The model under review builds one solid part; all positions refer to its coordinate system, in mm. Give positions to 0.01 mm unless a question says otherwise; leave off trailing zeros. Write each loop counter-clockwise with the first axis right and the second up, starting at its lowest first coordinate (ties: lowest second). Pieces come first, ordered by that corner, then holes. Notation, with made-up numbers: (75.5, -27) - (89.5, -27) arc R20 ccw to (89.5, -17) - close; hole circle Ø4 at (49, 53.25). An arc over 180 degrees is marked (long way). Write item = value, one per line.
```python
from build123d import *

# Parameters (mm, degrees)
F0_R     = 44.45
F1_DEPTH = 6.35
F3_DEPTH = 0.254


# Not quite as in the source:
# - ends of sketch curves that miss each other by under 0.0002 mm in the source are joined


with BuildPart() as f1:
    # F0 (on Top) → F1 (new body)
    with BuildSketch(Plane.XY):
        Circle(F0_R)
    extrude(amount=F1_DEPTH)

    # F2 (on face) → F3 (cut)
    with BuildSketch(Plane.XY.offset(6.35)):
        with BuildLine():
            Line((5.6039993651, 23.2917912652), (5.6039993651, 26.2641511811))
            Line((5.6039993651, 26.2641511811), (-3.5374157604, 26.2641511811))
            ThreePointArc((-3.5374157604, 26.2641511811), (-6.1724008767, 25.2877017598), (-7.2804156008, 22.7052797559))
            Line((-7.2804156008, 22.7052797559), (-7.2804156008, 14.3152289093))
            ThreePointArc((-7.2804156008, 14.3152289093), (-6.4557803762, 12.2478717336), (-4.4346582144, 11.3156409934))
            ThreePointArc((-4.4346582144, 11.3156409934), (1.3092272973, 11.2673019991), (7.0349466987, 11.7263169959))
            Line((7.0349466987, 11.7263169959), (7.0961336605, 12.2146336362))
            Line((7.0961336605, 12.2146336362), (7.0961336605, 19.8627323627))
            Line((7.0961336605, 19.8627323627), (0, 19.8627323627))
            Line((0, 19.8627323627), (0, 17.358450219))
            Line((0, 17.358450219), (2.9400843196, 17.3616167158))
            Line((2.9400843196, 17.3616167158), (2.9400843196, 14.1317071393))
            Line((2.9400843196, 14.1317071393), (0, 14.1317071393))
            Line((0, 14.1317071393), (-2.2346060723, 14.1317071393))
            ThreePointArc((-2.2346060723, 14.1317071393), (-2.7898678793, 14.3800667532), (-3.1146267429, 14.8943914101))
            ThreePointArc((-3.1146267429, 14.8943914101), (-3.2355914853, 15.5005322545), (-3.2674165577, 16.1178055789))
            Line((-3.2674165577, 16.1178055789), (-3.1592417437, 21.2145812126))
            ThreePointArc((-3.1592417437, 21.2145812126), (-3.1837866635, 21.575252567), (-3.1439608429, 21.9345577061))
            ThreePointArc((-3.1439608429, 21.9345577061), (-3.117530452, 22.198564373), (-3.1439608429, 22.4625710398))
            ThreePointArc((-3.1439608429, 22.4625710398), (-3.0817290753, 22.8241742068), (-2.7919525746, 23.0492502451))
            ThreePointArc((-2.7919525746, 23.0492502451), (-2.1422008965, 23.2306538656), (-1.4703774561, 23.2917912652))
            Line((-1.4703774561, 23.2917912652), (5.6039993651, 23.2917912652))
        make_face()
        with BuildLine():
            Line((-3.1592417437, 21.2145812126), (-3.1439608429, 21.9345577061))
            ThreePointArc((-3.1439608429, 21.9345577061), (-3.1837866635, 21.575252567), (-3.1592417437, 21.2145812126))
        make_face()
        Polygon((7.0961336605, 12.2146336362), (7.0349466987, 11.7263169959), (7.0961336605, 10.9925279394), (7.0961336605, 0.9659290663), (19.5016358048, 0.9659290663), (19.5016358048, 12.2146336362), align=None)
        Polygon((7.0961336605, 0.9659290663), (7.0961336605, 10.9925279394), (2.7143813204, 10.9925279394), (2.7143813204, 2.2997791572), (-2.7398910557, 10.9925279394), (-7.300500758, 10.9925279394), (-7.2804156008, 0), (-7.2804156008, -3.8537723012), (-6.2781353481, -3.8537723012), (-3.1410043308, -3.8537723012), (-3.1410043308, 4.7863919603), (2.6191033489, -3.8537723012), (7.0961336605, -3.8537723012), align=None)
        Polygon((-7.2804156008, 0), (-7.300500758, 10.9925279394), (-7.2804156008, 13.206558302), (-18.3086954057, 13.206558302), (-18.3086954057, 0), align=None)
        with BuildLine():
            Line((0, -7.2983574902), (6.6179535352, -7.2983574902))
            Line((6.6179535352, -7.2983574902), (6.6179535352, -4.2878086955))
            Line((6.6179535352, -4.2878086955), (-2.2489061664, -4.2878086955))
            ThreePointArc((-2.2489061664, -4.2878086955), (-4.0568875501, -4.6442817118), (-5.5942512015, -5.6603440615))
            ThreePointArc((-5.5942512015, -5.6603440615), (-6.1507192567, -6.4794007942), (-6.3533238135, -7.4486592847))
            Line((-6.3533238135, -7.4486592847), (-6.3533238135, -16.6105034737))
            ThreePointArc((-6.3533238135, -16.6105034737), (-5.8759308245, -17.9913268961), (-4.6476325952, -18.782440573))
            Line((-4.6476325952, -18.782440573), (-3.7075637703, -19.2863568686))
            Line((-3.7075637703, -19.2863568686), (3.3881619917, -19.303988614))
            Line((3.3881619917, -19.303988614), (6.6293859856, -18.9052186906))
            Line((6.6293859856, -18.9052186906), (6.593650474, -16.0276701207))
            Line((6.593650474, -16.0276701207), (0, -16.3928680122))
            ThreePointArc((0, -16.3928680122), (-0.7145080017, -16.4126398372), (-1.4290160034, -16.3928680122))
            ThreePointArc((-1.4290160034, -16.3928680122), (-2.080113152, -16.0523673946), (-2.251843689, -15.3379607946))
            Line((-2.251843689, -15.3379607946), (-2.251843689, -8.4599647671))
            ThreePointArc((-2.251843689, -8.4599647671), (-2.0899663646, -7.8730095416), (-1.6501033679, -7.4520092458))
            ThreePointArc((-1.6501033679, -7.4520092458), (-0.8286208401, -7.3368533365), (0, -7.2983574902))
        make_face()
        with BuildLine():
            Line((3.3881619917, -19.303988614), (-3.7075637703, -19.2863568686))
            Line((-3.7075637703, -19.2863568686), (-12.6563319936, -19.2641206086))
            Line((-12.6563319936, -19.2641206086), (-12.8377182409, -19.2641206086))
            Line((-12.8377182409, -19.2641206086), (-12.9873463884, -18.6591409147))
            ThreePointArc((-12.9873463884, -18.6591409147), (-13.1098010784, -17.8878071535), (-13.4031539783, -17.1640012413))
            ThreePointArc((-13.4031539783, -17.1640012413), (-13.5725884432, -16.8395453931), (-13.7304924428, -16.5093243122))
            ThreePointArc((-13.7304924428, -16.5093243122), (-14.0521811274, -16.0543913958), (-14.5178735256, -15.7484859228))
            ThreePointArc((-14.5178735256, -15.7484859228), (-15.086809482, -15.6747136098), (-15.6148988754, -15.8988833427))
            ThreePointArc((-15.6148988754, -15.8988833427), (-16.1466107031, -16.4449553577), (-16.5172908455, -17.1109195799))
            ThreePointArc((-16.5172908455, -17.1109195799), (-16.7501696159, -17.7330376736), (-16.9609729201, -18.3629784733))
            ThreePointArc((-16.9609729201, -18.3629784733), (-17.0934179213, -18.9312665088), (-17.1379111707, -19.5130854845))
            Line((-17.1379111707, -19.5130854845), (-17.1379111707, -19.8522191495))
            Line((-17.1379111707, -19.8522191495), (-19.3871874362, -19.8522191495))
            Line((-19.3871874362, -19.8522191495), (-19.3871874362, -22.8021256626))
            Line((-19.3871874362, -22.8021256626), (-17.0194374538, -22.8021256626))
            Line((-17.0194374538, -22.8021256626), (-17.0194374538, -23.2551640704))
            ThreePointArc((-17.0194374538, -23.2551640704), (-16.9093551317, -23.6838787474), (-16.7950224131, -24.1114795208))
            ThreePointArc((-16.7950224131, -24.1114795208), (-16.7338426372, -24.3328635786), (-16.6711639613, -24.5538279414))
            ThreePointArc((-16.6711639613, -24.5538279414), (-16.4738073507, -25.0326716474), (-16.1757338792, -25.4562199116))
            ThreePointArc((-16.1757338792, -25.4562199116), (-15.9267297619, -25.732701627), (-15.6729177634, -26.0047763574))
            ThreePointArc((-15.6729177634, -26.0047763574), (-14.9718242273, -26.3117655956), (-14.2623546636, -26.0246637372))
            ThreePointArc((-14.2623546636, -26.0246637372), (-13.7772653209, -25.4368959002), (-13.4154763073, -24.7661564499))
            ThreePointArc((-13.4154763073, -24.7661564499), (-13.2751868701, -24.4473909933), (-13.1237693131, -24.1337586194))
            ThreePointArc((-13.1237693131, -24.1337586194), (-12.9090296801, -23.5454392253), (-12.837051295, -22.9233042467))
            Line((-12.837051295, -22.9233042467), (-12.8377182409, -22.622095421))
            Line((-12.8377182409, -22.622095421), (0.5678676759, -22.592412358))
            Line((0.5678676759, -22.592412358), (12.5019904939, -22.6220667474))
            Line((12.5019904939, -22.6220667474), (12.5135298725, -22.622095421))
            Line((12.5135298725, -22.622095421), (12.6259239413, -22.622095421))
            Line((12.6259239413, -22.622095421), (12.6259239413, -22.8433404118))
            ThreePointArc((12.6259239413, -22.8433404118), (12.6900931034, -23.3765945805), (12.878936831, -23.8794024329))
            ThreePointArc((12.878936831, -23.8794024329), (13.1121897024, -24.7032143779), (13.6001783309, -25.4067341867))
            Line((13.6001783309, -25.4067341867), (13.7601625174, -25.5711600184))
            ThreePointArc((13.7601625174, -25.5711600184), (14.0077931702, -25.8774350672), (14.3499616533, -26.0724890977))
            ThreePointArc((14.3499616533, -26.0724890977), (14.8915415981, -26.1493664388), (15.4228175364, -26.0191172952))
            ThreePointArc((15.4228175364, -26.0191172952), (15.5930961418, -25.9161088082), (15.7359875739, -25.7775895298))
            ThreePointArc((15.7359875739, -25.7775895298), (16.5550328697, -24.4671777543), (17.0114282519, -22.9907911271))
            Line((17.0114282519, -22.9907911271), (17.0942133791, -22.5096959621))
            Line((17.0942133791, -22.5096959621), (19.0433021635, -22.5096959621))
            Line((19.0433021635, -22.5096959621), (19.0433021635, -19.4356404245))
            Line((19.0433021635, -19.4356404245), (17.0150939375, -19.4110530503))
            Line((17.0150939375, -19.4110530503), (17.0150939375, -19.0368138024))
            ThreePointArc((17.0150939375, -19.0368138024), (16.989674065, -18.7347053505), (16.9141292572, -18.4410922229))
            Line((16.9141292572, -18.4410922229), (16.690004617, -17.6846757531))
            ThreePointArc((16.690004617, -17.6846757531), (16.407642716, -17.0034564681), (15.9896202385, -16.3959655911))
            ThreePointArc((15.9896202385, -16.3959655911), (15.6603689447, -16.0642729564), (15.2857392253, -15.7848467735))
            ThreePointArc((15.2857392253, -15.7848467735), (14.6670179234, -15.6398096454), (14.0927875351, -15.9120435136))
            Line((14.0927875351, -15.9120435136), (13.9366754533, -16.0662262266))
            ThreePointArc((13.9366754533, -16.0662262266), (13.2239743808, -16.988100564), (12.7797400013, -18.0653428434))
            ThreePointArc((12.7797400013, -18.0653428434), (12.7644443964, -18.1246889663), (12.7497899169, -18.1841966471))
            ThreePointArc((12.7497899169, -18.1841966471), (12.6499744154, -18.7132948986), (12.6030528918, -19.2496776581))
            Line((12.6030528918, -19.2496776581), (12.6030528918, -19.3145554513))
            Line((12.6030528918, -19.3145554513), (9.0023325756, -19.3145554513))
            Line((9.0023325756, -19.3145554513), (3.3881619917, -19.303988614))
        make_face()
    extrude(amount=-F3_DEPTH, mode=Mode.SUBTRACT)


solid = f1.part
```
1. Insertion check: P1, Ø1, axis at x = 21, z = 3, coming from the -Y side; P2, Ø1.5, axis at y = 7.5, z = 1.5, coming from the -X side; P3, Ø1.5, axis at x = -23.5, z = 5.5, coming from the +Y side. Each pin has a flat end and moves straight along its axis. Give the tip position at first contact, or say it passes through.
Findings below:
P1 = -39.44
P2 = -43.93
P3 = 38.19
2. Draft analysis for pull direction X (two halves, no side actions). For faces 1 (the flat face through (-1, 1, 0)), 2 (the cylindrical face through (42.397, 13.352, 3.131)), 3 (the flat face through (0.3, 11.4, 6.096)), state which applies: +X half, -X half, draft (parallel to the pull), parting line (faces both ways), or undercut.
Findings below:
face_1 = draft
face_2 = parting line
face_3 = undercut
3. Take a section at B-B on x = -24.5. Give the boundary of the cut face in (y, z), and give its area (3 significant figures).
Findings below:
outline = (-37.09, 0) - (37.09, 0) - (37.09, 6.35) - (-37.09, 6.35) - close
area = 471 mm²
4. For line 1 (Z direction, x = 3.5, y = 25); line 2 (Y direction, x = 0, z = 0.5); line 3 (X direction, y = -9, z = 5), list the stretches that pass through material, from the lowest coordinate up. Write a range as from..to.
Findings below:
line_1 = 0..6.1
line_2 = -44.45..44.45
line_3 = -43.53..43.53
5. Take a section at A-A on z = 1. Give the boundary of the cut face in (x, y).
Findings below:
outline = circle Ø88.9 at (0, 0)
